The listing builds one solid part. Answer for the finished solid, in the listing's coordinates (mm). A direction names the side the tool comes from. Coordinates: 2 decimals unless noted, no trailing zeros. Loops run counter-clockwise (first coordinate to the right, second up) from the corner with the lowest first, then second, coordinate; pieces in that order, holes last. Notation, with made-up numbers: (48, 50) - (107, 50) arc R18 ccw to (107, 77) - close; hole circle Ø5 at (30.25, 68). An arc over 180 degrees is marked (long way). Return JSON: item names as keys, results as strings. Group by question number.
1. Find the intervals of material crossed by line 1 along X through (y, z) = (2.75, 22.5); line 2 along Y through (x, z) = (-1.5, 4.5); line 3 along Y through (x, z) = (-0.5, 25), in increasing order.
2. Which of the six approach directions +Z, -Z, +X, -X, +Y, -Y give full straight-line access (tool end or side, diameter ignored) to faces 1 (the face through (3, 12, 3)), 2 (the face through (41.301, 8.718, 30.355)), 3 (the face through (47, 3, 23))?
3. Each of these flat-tipped pins is pushed along its axis until it touches: P1, Ø2.5, axis at y = 9, z = 5.5, coming from the -X side; P2, Ø3, axis at y = 13, z = 34.5, coming from the +X side; P3, Ø13.5, axis at x = 9.5, z = 32, coming from the +Y side. Where does it stop, or does it pass through?
4. Section B-B (y = 3.5) is taken. Write down the section's boundary in (x, z).
5. Section D-D (z = 30) is taken. Write down the section's boundary in (x, y), and give its area (3 significant figures).
6. Section A-A (y = 14.5) is taken. State how many separate pieces and enclosed holes the cut face has, and give its area (3 significant figures).
7. The mould has two halves that part along X. Classify faces 4 (the face through (38.98, 11.43, 34.13)), 5 (the face through (41.2, 11, 30.2)), 6 (the face through (18, 3, 0.5)), 7 (the face through (-10, 9, 15)): pulls with the +X half, pulls with the -X half, needs draft (parallel to the pull), parting line crosses it, or undercut.
8. Section C-C (z = 22.5) is taken. Write down the section's boundary in (x, y), and give its area (3 significant figures).
```python
from build123d import *

# Parameters (mm, degrees)
SKETCH_1_R          = 1.75
SKETCH_1_W          = 20
SKETCH_1_H          = 8.5
EXTRUDE_1_DEPTH     = 7
EXTRUDE_2_DEPTH     = 17
EXTRUDE_3_DEPTH     = 11
SKETCH_1_4_W        = 20
SKETCH_1_4_H        = 8.5
EXTRUDE_4_DEPTH     = 12
SHELL_START         = 0.5
SHELL_4_OUTLINE_R   = 2.25
SHELL_4_DEPTH       = 6
SHELL_START_2       = 6.5
SHELL_4_2_DEPTH     = 10
SHELL_4_3_OUTLINE_W = 19
SHELL_4_3_OUTLINE_H = 8
SHELL_4_3_DEPTH     = 5


# Read off the part's stored shape, not the designer's step: 抽壳4
with BuildPart() as part:
    # 草图1 → 凸台-拉伸1 (new body)
    with BuildSketch(Plane(origin=(0, 0, 0), x_dir=(1, 0, 0), z_dir=(0, 1, 0))):
        Polygon((0, 0), (35, 0), (47.5, -12.5), (47.5, -32.5), (35, -45), (0, -45), (-12.5, -32.5), (-12.5, -12.5), align=None)
        with Locations(Location((33.75, -22.5, 0), (0, 0, 270))):
            Circle(SKETCH_1_R, mode=Mode.SUBTRACT)
        with Locations(Location((1.25, -22.5, 0), (0, 0, 90))):
            Circle(SKETCH_1_R, mode=Mode.SUBTRACT)
        Polygon((33.585786438, -43.585786438), (41.363961031, -35.807611845), (37.2627417, -31.706392514), (29.484567107, -39.484567107), align=None, mode=Mode.SUBTRACT)
        Polygon((46.085786438, -31.085786438), (41.984567107, -35.187005769), (38.87329727, -32.075735931), (42.9745166, -27.9745166), align=None, mode=Mode.SUBTRACT)
        Polygon((33.585786438, -1.414213562), (41.363961031, -9.192388155), (37.2627417, -13.293607486), (29.484567107, -5.515432893), align=None, mode=Mode.SUBTRACT)
        Polygon((46.085786438, -13.914213562), (41.984567107, -9.812994231), (38.87329727, -12.924264069), (42.9745166, -17.0254834), align=None, mode=Mode.SUBTRACT)
        Polygon((-7.9745166, -17.0254834), (-11.085786438, -13.914213562), (-6.984567107, -9.812994231), (-3.87329727, -12.924264069), align=None, mode=Mode.SUBTRACT)
        Polygon((5.515432893, -5.515432893), (1.414213562, -1.414213562), (-6.363961031, -9.192388155), (-2.2627417, -13.293607486), align=None, mode=Mode.SUBTRACT)
        Polygon((-11.085786438, -31.085786438), (-6.984567107, -35.187005769), (-3.87329727, -32.075735931), (-7.9745166, -27.9745166), align=None, mode=Mode.SUBTRACT)
        Polygon((-6.363961031, -35.807611845), (-2.2627417, -31.706392514), (5.515432893, -39.484567107), (1.414213562, -43.585786438), align=None, mode=Mode.SUBTRACT)
        with Locations((17.5, -6.25)):
            Rectangle(SKETCH_1_W, SKETCH_1_H, mode=Mode.SUBTRACT)
    extrude(amount=EXTRUDE_1_DEPTH)

    # 草图1<2> → 凸台-拉伸2 (add)
    with BuildSketch(Plane(origin=(0, 0, 0), x_dir=(1, 0, 0), z_dir=(0, 1, 0))):
        Polygon((37.2627417, -13.293607486), (29.484567107, -5.515432893), (33.585786438, -1.414213562), (41.363961031, -9.192388155), align=None)
        Polygon((-6.363961031, -9.192388155), (-2.2627417, -13.293607486), (5.515432893, -5.515432893), (1.414213562, -1.414213562), align=None)
        Polygon((-2.2627417, -31.706392514), (5.515432893, -39.484567107), (1.414213562, -43.585786438), (-6.363961031, -35.807611845), align=None)
        Polygon((37.2627417, -31.706392514), (29.484567107, -39.484567107), (33.585786438, -43.585786438), (41.363961031, -35.807611845), align=None)
    extrude(amount=EXTRUDE_2_DEPTH)

    # 草图1<3> → 凸台-拉伸3 (add)
    with BuildSketch(Plane(origin=(0, 0, 0), x_dir=(1, 0, 0), z_dir=(0, 1, 0))):
        Polygon((-11.085786438, -31.085786438), (-6.984567107, -35.187005769), (-3.87329727, -32.075735931), (-7.9745166, -27.9745166), align=None)
        Polygon((42.9745166, -27.9745166), (46.085786438, -31.085786438), (41.984567107, -35.187005769), (38.87329727, -32.075735931), align=None)
        Polygon((41.984567107, -9.812994231), (38.87329727, -12.924264069), (42.9745166, -17.0254834), (46.085786438, -13.914213562), align=None)
        Polygon((-6.984567107, -9.812994231), (-3.87329727, -12.924264069), (-7.9745166, -17.0254834), (-11.085786438, -13.914213562), align=None)
    extrude(amount=EXTRUDE_3_DEPTH)

    # 草图1<4> → 凸台-拉伸4 (add)
    with BuildSketch(Plane(origin=(0, 0, 0), x_dir=(1, 0, 0), z_dir=(0, 1, 0))):
        with Locations((17.5, -6.25)):
            Rectangle(SKETCH_1_4_W, SKETCH_1_4_H)
    extrude(amount=EXTRUDE_4_DEPTH)

    # 抽壳4 outline → 抽壳4 (cut)
    with BuildSketch(Plane(origin=(0, 0, 0), x_dir=(1, 0, 0), z_dir=(0, 1, 0)).offset(SHELL_START)):
        Polygon((0.207106781, -0.5), (-12, -12.707106781), (-12, -32.292893219), (0.207106781, -44.5), (34.792893219, -44.5), (47, -32.292893219), (47, -12.707106781), (34.792893219, -0.5), align=None)
        with Locations((1.25, -22.5)):
            Circle(SHELL_4_OUTLINE_R, mode=Mode.SUBTRACT)
        with Locations((33.75, -22.5)):
            Circle(SHELL_4_OUTLINE_R, mode=Mode.SUBTRACT)
    extrude(amount=SHELL_4_DEPTH, mode=Mode.SUBTRACT)

    # Shell 4 2 outline → Shell 4 2 (cut)
    with BuildSketch(Plane(origin=(0, 0, 0), x_dir=(1, 0, 0), z_dir=(0, 1, 0)).offset(SHELL_START_2)):
        Polygon((33.585786438, -2.121320344), (30.191673888, -5.515432893), (37.2627417, -12.586500705), (40.656854249, -9.192388155), align=None)
        Polygon((45.378679656, -13.914213562), (41.984567107, -10.520101013), (39.580404051, -12.924264069), (42.9745166, -16.318376618), align=None)
        Polygon((-5.656854249, -9.192388155), (-2.2627417, -12.586500705), (4.808326112, -5.515432893), (1.414213562, -2.121320344), align=None)
        Polygon((-4.580404051, -12.924264069), (-6.984567107, -10.520101013), (-10.378679656, -13.914213562), (-7.9745166, -16.318376618), align=None)
        Polygon((4.808326112, -39.484567107), (-2.2627417, -32.413499295), (-5.656854249, -35.807611845), (1.414213562, -42.878679656), align=None)
        Polygon((-10.378679656, -31.085786438), (-6.984567107, -34.479898987), (-4.580404051, -32.075735931), (-7.9745166, -28.681623382), align=None)
        Polygon((37.2627417, -32.413499295), (30.191673888, -39.484567107), (33.585786438, -42.878679656), (40.656854249, -35.807611845), align=None)
        Polygon((39.580404051, -32.075735931), (41.984567107, -34.479898987), (45.378679656, -31.085786438), (42.9745166, -28.681623382), align=None)
    extrude(amount=SHELL_4_2_DEPTH, mode=Mode.SUBTRACT)

    # Shell 4 3 outline → Shell 4 3 (cut)
    with BuildSketch(Plane(origin=(0, 0, 0), x_dir=(1, 0, 0), z_dir=(0, 1, 0)).offset(SHELL_START_2)):
        with Locations((17.5, -6)):
            Rectangle(SHELL_4_3_OUTLINE_W, SHELL_4_3_OUTLINE_H)
    extrude(amount=SHELL_4_3_DEPTH, mode=Mode.SUBTRACT)


solid = part.part
```
The answers:
{
 "1": {"line 1": "x = -12.5 to -12, -1 to -0.5, 3 to 3.5, 31.5 to 32, 35.5 to 36, 47 to 47.5", "line 2": "y = 0 to 0.5, 6.5 to 17", "line 3": "y = 0 to 0.5, 6.5 to 7"},
 "2": {"face 1": "-Z, +Y", "face 2": "+Y", "face 3": "none"},
 "3": {"P1": "stops at x = -3.92", "P2": "stops at x = 41.36", "P3": "stops at y = 7"},
 "4": {"outline": "(-12.5, 12.5) - (0, 0) - (35, 0) - (47.5, 12.5) - (47.5, 32.5) - (35, 45) - (0, 45) - (-12.5, 32.5) - close; circle Ø4.5 at (1.25, 22.5); circle Ø4.5 at (33.75, 22.5); hole (-12, 12.71) - (0.21, 0.5) - (34.79, 0.5) - (47, 12.71) - (47, 32.29) - (34.79, 44.5) - (0.21, 44.5) - (-12, 32.29) - close; hole circle Ø3.5 at (1.25, 22.5); hole circle Ø3.5 at (33.75, 22.5)"},
 "5": {"outline": "(-12.5, 0) - (47.5, 0) - (47.5, 7) - (45, 7) - (45, 11) - (44.29, 11) - (44.29, 6.5) - (47, 6.5) - (47, 0.5) - (-12, 0.5) - (-12, 6.5) - (-9.29, 6.5) - (-9.29, 11) - (-10, 11) - (-10, 7) - (-12.5, 7) - close; (-6.66, 6.5) - (41.66, 6.5) - (41.66, 11) - (40.95, 11) - (40.95, 7) - (-5.95, 7) - (-5.95, 11) - (-6.66, 11) - close", "area": "74.7 mm2"},
 "6": {"separate pieces": "4", "enclosed holes": "4", "area": "63.2 mm2"},
 "7": {"face 4": "undercut", "face 5": "needs draft", "face 6": "undercut", "face 7": "pulls with the -X half"},
 "8": {"outline": "(-12.5, 0) - (-0.5, 0) - (-0.5, 7) - (-12.5, 7) - close; (3, 0) - (32, 0) - (32, 7) - (3, 7) - close; (35.5, 0) - (47.5, 0) - (47.5, 7) - (35.5, 7) - close; hole (-12, 0.5) - (-1, 0.5) - (-1, 6.5) - (-12, 6.5) - close; hole (3.5, 0.5) - (31.5, 0.5) - (31.5, 6.5) - (3.5, 6.5) - close; hole (36, 0.5) - (47, 0.5) - (47, 6.5) - (36, 6.5) - close", "area": "71.0 mm2"}
}
